Print and shaded views of the part. All mm, measured from the part's lowest x, y and z. A direction names the side the tool comes from. Coordinates: 2 decimals unless noted, no trailing zeros. Write each loop counter-clockwise with the first axis right and the second up, starting at its lowest first coordinate (ties: lowest second). Pieces come first, ordered by that corner, then holes. Notation, with made-up numbers: (28.25, -38) -> (63.25, -38) arc R21 cw to (63.25, -20) -> close; hole circle Ø8 at (46, 89.25). An arc over 180 degrees is marked (long way). Write item = value, one per line.
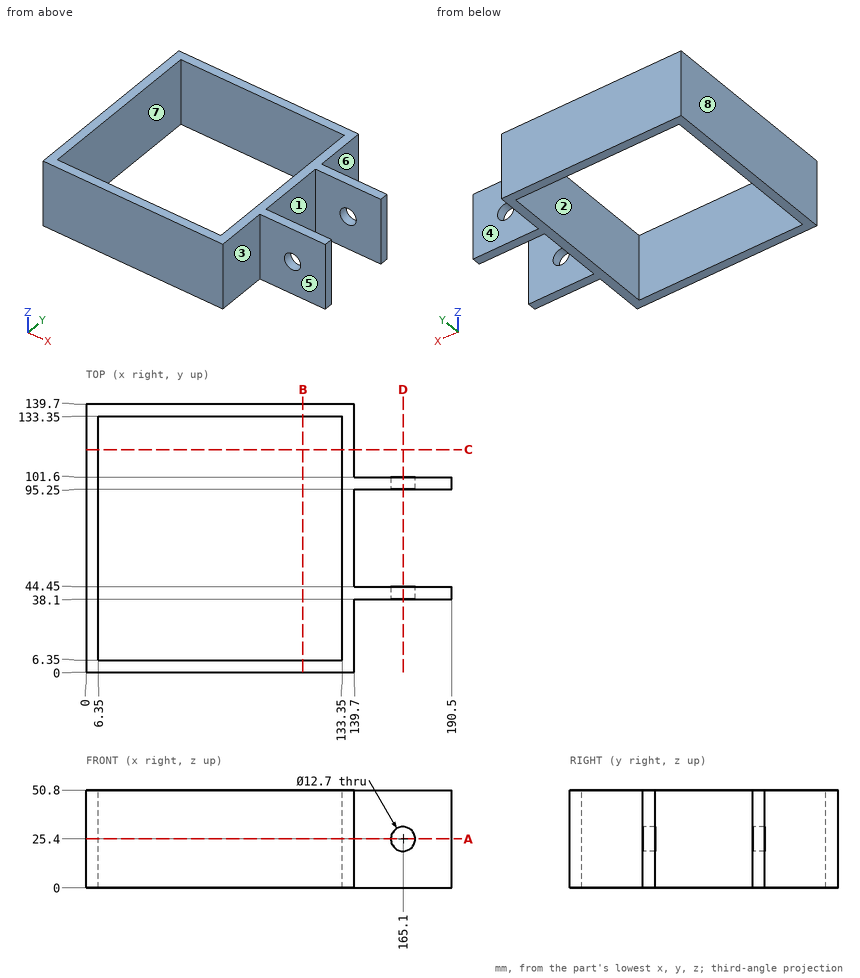
Q1. Saw through at A-A on z = 25.4. Give the cut face in (x, y), and give its area (3 significant figures).
Model answer:
outline = (0, 0) -> (139.7, 0) -> (139.7, 38.1) -> (158.75, 38.1) -> (158.75, 44.45) -> (139.7, 44.45) -> (139.7, 95.25) -> (158.75, 95.25) -> (158.75, 101.6) -> (139.7, 101.6) -> (139.7, 139.7) -> (0, 139.7) -> close; (171.45, 38.1) -> (190.5, 38.1) -> (190.5, 44.45) -> (171.45, 44.45) -> close; (171.45, 95.25) -> (190.5, 95.25) -> (190.5, 101.6) -> (171.45, 101.6) -> close; hole (6.35, 6.35) -> (133.35, 6.35) -> (133.35, 133.35) -> (6.35, 133.35) -> close
area = 3,870 mm²
Q2. Saw through at B-B on x = 113. Give the cut face in (y, z).
Model answer:
outline = (0, 0) -> (6.35, 0) -> (6.35, 50.8) -> (0, 50.8) -> close; (133.35, 0) -> (139.7, 0) -> (139.7, 50.8) -> (133.35, 50.8) -> close
Q3. Probe line 1 (X direction, y = 41, z = 25); line 2 (X direction, y = 52, z = 22.5). List the from-to ranges inside material, lowest first. Write a range as from..to.
Model answer:
line_1 = 0..6.35, 133.35..158.76, 171.44..190.5
line_2 = 0..6.35, 133.35..139.7
Q4. Pin check, flat tips, straight feed: pin 1 (14.5 mm diameter, centred on x = 165.1, z = 25.4, fed in from +Y); pin 2 (7.5 mm diameter, centred on x = 165.1, z = 25.4, fed in from +Y); pin 3 (15 mm diameter, centred on x = 161, z = 29.5, fed in from -Y); pin 4 (11.5 mm diameter, centred on y = 18, z = 29, fed in from +X). Stop position of each tip, or through.
Model answer:
pin_1 = 101.6
pin_2 = through
pin_3 = 38.1
pin_4 = 139.7
Q5. Mould opens along X. For the marked faces 5, 6, 7 and 8 say: released by +X, released by -X, zero draft, split by the parting line, or undercut.
Model answer:
face_5 = zero draft
face_6 = released by +X
face_7 = undercut
face_8 = released by -X
Q6. Saw through at D-D on x = 165.1. Give the cut face in (y, z).
Model answer:
outline = (38.1, 0) -> (44.45, 0) -> (44.45, 19.05) -> (38.1, 19.05) -> close; (38.1, 31.75) -> (44.45, 31.75) -> (44.45, 50.8) -> (38.1, 50.8) -> close; (95.25, 0) -> (101.6, 0) -> (101.6, 19.05) -> (95.25, 19.05) -> close; (95.25, 31.75) -> (101.6, 31.75) -> (101.6, 50.8) -> (95.25, 50.8) -> close
Q7. Which spindle directions (+Z, -Z, +X, -X, +Y, -Y) get a long thin tool onto all of the face, cutting with end or side? Do the marked faces 1, 2, 3 and 4. Say none if no direction does.
Model answer:
face_1 = +Z, -Z, +X
face_2 = +Z, -Z
face_3 = +Z, -Z, +X, -Y
face_4 = +Z, -Z, +X, +Y
